Work out the finished part from the listing and answer in its coordinate system (mm). A direction names the side the tool comes from. Give positions to 0.01 mm unless a question says otherwise; leave off trailing zeros. Put each result on its own line as item: value.
```python
from build123d import *

# Parameters (mm, degrees)
SKETCH1_R                       = 2.25
BOSS_EXTRUDE1_DEPTH             = 12.7
TAP_DRILL_FOR_M6X1_0_TAP1_D     = 5
TAP_DRILL_FOR_M6X1_0_TAP1_DEPTH = 17
TAP_DRILL_FOR_M6X1_0_TAP1_TIP   = 1.502151548
F_6_0MM_DOWEL_HOLE1_D           = 6
F_6_0MM_DOWEL_HOLE1_DEPTH       = 17
F_6_0MM_DOWEL_HOLE1_TIP         = 1.802581857


with BuildPart() as part:
    # Sketch1 → Boss-Extrude1 (new body)
    with BuildSketch(Plane(origin=(0, 0, 0), x_dir=(1, 0, 0), z_dir=(0, 1, 0))):
        with BuildLine():
            Line((48.34884719, 117.5), (48.34884719, -117.5))
            Line((48.34884719, -117.5), (-21.65115281, -117.5))
            ThreePointArc((-21.65115281, -117.5), (-28.722220622, -114.571067812), (-31.65115281, -107.5))
            Line((-31.65115281, -107.5), (-31.65115281, 107.5))
            ThreePointArc((-31.65115281, 107.5), (-28.722220622, 114.571067812), (-21.65115281, 117.5))
            Line((-21.65115281, 117.5), (48.34884719, 117.5))
        make_face()
        with Locations(Location((-16.17615281, -97.5, 0), (0, 0, 270))):
            Circle(SKETCH1_R, mode=Mode.SUBTRACT)
        with Locations(Location((13.82384719, -97.5, 0), (0, 0, 270))):
            Circle(SKETCH1_R, mode=Mode.SUBTRACT)
        with Locations(Location((13.82384719, -72.5, 0), (0, 0, 270))):
            Circle(SKETCH1_R, mode=Mode.SUBTRACT)
        with Locations(Location((-16.17615281, -72.5, 0), (0, 0, 270))):
            Circle(SKETCH1_R, mode=Mode.SUBTRACT)
        with Locations(Location((-16.17615281, 72.5, 0), (0, 0, 270))):
            Circle(SKETCH1_R, mode=Mode.SUBTRACT)
        with Locations(Location((-16.17615281, 97.5, 0), (0, 0, 270))):
            Circle(SKETCH1_R, mode=Mode.SUBTRACT)
        with Locations(Location((13.82384719, 97.5, 0), (0, 0, 270))):
            Circle(SKETCH1_R, mode=Mode.SUBTRACT)
        with Locations(Location((13.82384719, 72.5, 0), (0, 0, 270))):
            Circle(SKETCH1_R, mode=Mode.SUBTRACT)
    extrude(amount=BOSS_EXTRUDE1_DEPTH)

    # Tap Drill for M6x1.0 Tap1
    with Locations(Plane(origin=(48.34884719, 0, 0), x_dir=(0, 0, -1), z_dir=(1, 0, 0))):
        with Locations((-100, 6.35), (-50, 6.35), (0, 6.35), (50, 6.35), (100, 6.35)):
            Hole(TAP_DRILL_FOR_M6X1_0_TAP1_D / 2, depth=TAP_DRILL_FOR_M6X1_0_TAP1_DEPTH)
            with Locations((0, 0, -(TAP_DRILL_FOR_M6X1_0_TAP1_DEPTH + TAP_DRILL_FOR_M6X1_0_TAP1_TIP / 2))):  # 118° drill point
                Cone(0, TAP_DRILL_FOR_M6X1_0_TAP1_D / 2, TAP_DRILL_FOR_M6X1_0_TAP1_TIP, mode=Mode.SUBTRACT)

    # Ø6.0mm Dowel Hole1
    with Locations(Plane(origin=(48.34884719, 0, 0), x_dir=(0, 0, -1), z_dir=(1, 0, 0))):
        with Locations((-75, 6.35), (75, 6.35)):
            Hole(F_6_0MM_DOWEL_HOLE1_D / 2, depth=F_6_0MM_DOWEL_HOLE1_DEPTH)
            with Locations((0, 0, -(F_6_0MM_DOWEL_HOLE1_DEPTH + F_6_0MM_DOWEL_HOLE1_TIP / 2))):  # 118° drill point
                Cone(0, F_6_0MM_DOWEL_HOLE1_D / 2, F_6_0MM_DOWEL_HOLE1_TIP, mode=Mode.SUBTRACT)


solid = part.part
```
(1) A tool of negligible diameter and unlimited length cuts with its end or side. For faces 4 (the face through (-15.5, 6.261, 99.646)), 5 (the face through (39.73, 8.83, -0.33)), from which of +Z, -Z, +X, -X, +Y, -Y can it reach the whole face along a straight path? Write none if from no direction.
Geometry check:
face 4: +Y, -Y
face 5: +X
(2) Given pin 1 (4.5 mm diameter, centred on y = 6.35, z = 100, fed in from +X); pin 2 (3 mm diameter, centred on y = 6.35, z = -50, fed in from +X), each flat-ended and moving along its own axis, determine where each tip first touches the part or whether it passes through.
Geometry check:
pin 1: stops at x = 31.2
pin 2: stops at x = 30.75
(3) Determine the mould class of faces 1 (the face through (12.962, 6.261, -95.422)), 2 (the face through (9, 0, -2)), 3 (the face through (14, 6, 117.5)) for opening direction Z: pulls with the +Z half, pulls with the -Z half, needs draft (parallel to the pull), parting line crosses it, or undercut.
Geometry check:
face 1: undercut
face 2: needs draft
face 3: pulls with the +Z half
(4) Straight lines are drawn through the part: line 1 (X direction, y = 7.25, z = -97.5); line 2 (Y direction, x = 35, z = -50); line 3 (Y direction, x = 36, z = -75). For each, find the intervals that lie inside material, in ascending order.
Geometry check:
line 1: x = -31.65 to -18.43, -13.93 to 11.57, 16.07 to 48.35
line 2: y = 0 to 3.85, 8.85 to 12.7
line 3: y = 0 to 3.35, 9.35 to 12.7
